from build123d import *

# Parameters (mm, degrees)
SKETCH_1_W                        = 240
SKETCH_1_H                        = 125
EXTRUDE_1_DEPTH                   = 4
HOLE_WIZARD_5_4_5_4_1_D           = 5.4
HOLE_WIZARD_5_4_5_4_1_CSINK_D     = 5.45
HOLE_WIZARD_5_4_5_4_1_CSINK_ANGLE = 90
FILLET_1_R                        = 3
SKETCH_4_R                        = 10
EXTRUDE_2_DEPTH                   = 6
SKETCH_6_W                        = 6.5
SKETCH_6_H                        = 20
EXTRUDE_3_DEPTH                   = 8
SKETCH_7_R                        = 2
CUT_EXTRUDE_1_DEPTH               = 14
FILLET_2_R                        = 4
FILLET_3_R                        = 4
FILLET_4_R                        = 4
EXTRUDE_START                     = 23.5
EXTRUDE_4_DEPTH                   = 8
SKETCH_9_R                        = 5.5
EXTRUDE_5_DEPTH                   = 5
FILLET_5_R                        = 4
FILLET_6_R                        = 4
SKETCH_12_W                       = 7
SKETCH_12_H                       = 8
EXTRUDE_6_DEPTH                   = 20
CUT_EXTRUDE_2_REACH               = 161.108
SKETCH_13_R                       = 2.1
EXTRUDE_7_DEPTH                   = 80
SKETCH_15_R                       = 2.5
EXTRUDE_8_DEPTH                   = 4
EXTRUDE_START_2                   = 15
SKETCH_17_R                       = 2.5
EXTRUDE_9_DEPTH                   = 15


with BuildPart() as part:
    # 草图1 → 凸台-拉伸1 (new body)
    with BuildSketch(Plane(origin=(0, 0, 0), x_dir=(1, 0, 0), z_dir=(0, 1, 0))):
        Rectangle(SKETCH_1_W, SKETCH_1_H)
    extrude(amount=EXTRUDE_1_DEPTH)

    # Ø5.4 (5.4) 直径孔1 (through all)
    with Locations(Plane(origin=(0, 4, 0), x_dir=(1, 0, 0), z_dir=(0, 1, 0))):
        with Locations((112, 54.5), (-112, 54.5), (-112, -54.5), (112, -54.5)):
            CounterSinkHole(HOLE_WIZARD_5_4_5_4_1_D / 2, HOLE_WIZARD_5_4_5_4_1_CSINK_D / 2, counter_sink_angle=HOLE_WIZARD_5_4_5_4_1_CSINK_ANGLE)

    # 圆角1
    fillet_1_edges = [part.edges().sort_by_distance(p)[0] for p in [
        (120, 2, 62.5),
        (-120, 2, 62.5),
        (-120, 2, -62.5),
        (120, 2, -62.5),
    ]]
    fillet(fillet_1_edges, radius=FILLET_1_R)

    # 草图4 → 凸台-拉伸2 (add)
    with BuildSketch(Plane.XY):
        with BuildLine():
            Line((-100, 4), (-46, 4))
            Line((-46, 4), (-46, 36))
            Line((-46, 36), (-73.452041029, 36))
            ThreePointArc((-73.452041029, 36), (-83.25, 40), (-93.047958971, 36))
            Line((-93.047958971, 36), (-100, 36))
            Line((-100, 36), (-100, 4))
        make_face()
        with Locations((-83.25, 26)):
            Circle(SKETCH_4_R, mode=Mode.SUBTRACT)
    extrude(amount=EXTRUDE_2_DEPTH)

    # 草图6 → 凸台-拉伸3 (add)
    with BuildSketch(Plane.XY.offset(6)):
        with Locations((-96.75, 26)):
            Rectangle(SKETCH_6_W, SKETCH_6_H)
        with Locations((-49.25, 26)):
            Rectangle(SKETCH_6_W, SKETCH_6_H)
    extrude(amount=EXTRUDE_3_DEPTH)

    # 草图7 → 切除-拉伸1 (cut)
    with BuildSketch(Plane.XY.offset(14)):
        with Locations((-96.75, 31)):
            Circle(SKETCH_7_R)
        with Locations((-96.75, 21)):
            Circle(SKETCH_7_R)
        with Locations((-49.25, 21)):
            Circle(SKETCH_7_R)
        with Locations((-49.25, 31)):
            Circle(SKETCH_7_R)
    extrude(amount=-CUT_EXTRUDE_1_DEPTH, mode=Mode.SUBTRACT)

    # 圆角2
    fillet_2_edges = [part.edges().sort_by_distance(p)[0] for p in [
        (-49.25, 16, 6),
        (-96.75, 16, 6),
    ]]
    fillet(fillet_2_edges, radius=FILLET_2_R)

    # 圆角3
    fillet_3_edges = [part.edges().sort_by_distance(p)[0] for p in [
        (-73, 4, 6),
    ]]
    fillet(fillet_3_edges, radius=FILLET_3_R)

    # 圆角4
    fillet_4_edges = [part.edges().sort_by_distance(p)[0] for p in [
        (-73, 4, 0),
        (-100, 4, 5),
        (-46, 4, 5),
    ]]
    fillet(fillet_4_edges, radius=FILLET_4_R)

    # 草图8 → 凸台-拉伸4 (add)
    with BuildSketch(Plane(origin=(0, 0, 0), x_dir=(-1, 0, 0), z_dir=(0, 0, -1)).offset(EXTRUDE_START)):
        with BuildLine():
            Line((73, 8), (73, 36))
            ThreePointArc((73, 36), (83.25, 40), (93.5, 36))
            Line((93.5, 36), (93.5, 8))
            Line((93.5, 8), (93.5, 4))
            Line((93.5, 4), (73, 4))
            Line((73, 4), (73, 8))
        make_face()
    extrude(amount=EXTRUDE_4_DEPTH)

    # 草图9 → 凸台-拉伸5 (add)
    with BuildSketch(Plane.XY.offset(-23.5)):
        with Locations((-83.116793534, 25.812971514)):
            Circle(SKETCH_9_R)
    extrude(amount=EXTRUDE_5_DEPTH)

    # 圆角5
    fillet_5_edges = [part.edges().sort_by_distance(p)[0] for p in [
        (-83.25, 4, -31.5),
    ]]
    fillet(fillet_5_edges, radius=FILLET_5_R)

    # 圆角6
    fillet_6_edges = [part.edges().sort_by_distance(p)[0] for p in [
        (-73, 4, -29.5),
        (-83.25, 4, -23.5),
        (-93.5, 4, -29.5),
    ]]
    fillet(fillet_6_edges, radius=FILLET_6_R)

    # 草图12 → 凸台-拉伸6 (add)
    with BuildSketch(Plane(origin=(0, 4, 0), x_dir=(1, 0, 0), z_dir=(0, 1, 0))):
        with Locations((116.5, -30.016568117)):
            Rectangle(SKETCH_12_W, SKETCH_12_H)
        with Locations((69.5, -30.016568117)):
            Rectangle(SKETCH_12_W, SKETCH_12_H)
    extrude(amount=EXTRUDE_6_DEPTH)

    # 草图13 → 切除-拉伸2 (cut, up to next)
    with BuildSketch(Plane.XY.offset(34.016568117), mode=Mode.PRIVATE) as cut_extrude_2_sk1:
        with Locations((69.5, 19)):
            Circle(SKETCH_13_R)
    cut_extrude_2_tool1 = extrude(cut_extrude_2_sk1.sketch, amount=-CUT_EXTRUDE_2_REACH, mode=Mode.PRIVATE) & part.part
    # 草图13 → 切除-拉伸2 (cut, up to next)
    with BuildSketch(Plane.XY.offset(34.016568117), mode=Mode.PRIVATE) as cut_extrude_2_sk2:
        with Locations((69.5, 9)):
            Circle(SKETCH_13_R)
    cut_extrude_2_tool2 = extrude(cut_extrude_2_sk2.sketch, amount=-CUT_EXTRUDE_2_REACH, mode=Mode.PRIVATE) & part.part
    # 草图13 → 切除-拉伸2 (cut, up to next)
    with BuildSketch(Plane.XY.offset(34.016568117), mode=Mode.PRIVATE) as cut_extrude_2_sk3:
        with Locations((116.5, 9)):
            Circle(SKETCH_13_R)
    cut_extrude_2_tool3 = extrude(cut_extrude_2_sk3.sketch, amount=-CUT_EXTRUDE_2_REACH, mode=Mode.PRIVATE) & part.part
    # 草图13 → 切除-拉伸2 (cut, up to next)
    with BuildSketch(Plane.XY.offset(34.016568117), mode=Mode.PRIVATE) as cut_extrude_2_sk4:
        with Locations((116.5, 19)):
            Circle(SKETCH_13_R)
    cut_extrude_2_tool4 = extrude(cut_extrude_2_sk4.sketch, amount=-CUT_EXTRUDE_2_REACH, mode=Mode.PRIVATE) & part.part
    add(cut_extrude_2_tool1.solids().sort_by_distance((69.5, 19, 34.016568))[0], mode=Mode.SUBTRACT)
    add(cut_extrude_2_tool2.solids().sort_by_distance((69.5, 9, 34.016568))[0], mode=Mode.SUBTRACT)
    add(cut_extrude_2_tool3.solids().sort_by_distance((116.5, 9, 34.016568))[0], mode=Mode.SUBTRACT)
    add(cut_extrude_2_tool4.solids().sort_by_distance((116.5, 19, 34.016568))[0], mode=Mode.SUBTRACT)

    # 草图14 → 凸台-拉伸7 (add)
    with BuildSketch(Plane(origin=(0, 4, 0), x_dir=(1, 0, 0), z_dir=(0, 1, 0))):
        with BuildLine():
            Line((109.3, -51.016568117), (96.7, -51.016568117))
            Line((96.7, -51.016568117), (-31.378587674, -51.016568117))
            Line((-31.378587674, -51.016568117), (-31.378587674, 51.016568117))
            Line((-31.378587674, 51.016568117), (95.460915007, 51.016568117))
            Line((95.460915007, 51.016568117), (96.7, 51.016568117))
            Line((96.7, 51.016568117), (109.3, 51.016568117))
            Line((109.3, 51.016568117), (109.3, 54.131727003))
            ThreePointArc((109.3, 54.131727003), (109.275, 54.5), (109.3, 54.868272997))
            Line((109.3, 54.868272997), (109.3, 57.016568117))
            Line((109.3, 57.016568117), (-37.378587674, 57.016568117))
            Line((-37.378587674, 57.016568117), (-37.378587674, -50.764100258))
            Line((-37.378587674, -50.764100258), (-37.378587674, -57.016568117))
            Line((-37.378587674, -57.016568117), (109.3, -57.016568117))
            Line((109.3, -57.016568117), (109.3, -54.868272997))
            ThreePointArc((109.3, -54.868272997), (109.275, -54.5), (109.3, -54.131727003))
            Line((109.3, -54.131727003), (109.3, -51.016568117))
        make_face()
    extrude(amount=EXTRUDE_7_DEPTH)

    # 草图15 → 凸台-拉伸8 (add)
    with BuildSketch(Plane(origin=(0, 0, 51.016568117), x_dir=(-1, 0, 0), z_dir=(0, 0, -1))):
        with Locations((-103, 14)):
            Circle(SKETCH_15_R)
    extrude(amount=EXTRUDE_8_DEPTH)

    # 草图17 → 凸台-拉伸9 (add)
    with BuildSketch(Plane.XY.offset(-51.016568117).offset(EXTRUDE_START_2)):
        with Locations(Location((103, 14, 0), (0, 0, 180))):
            Circle(SKETCH_17_R)
    extrude(amount=-EXTRUDE_9_DEPTH)


solid = part.part
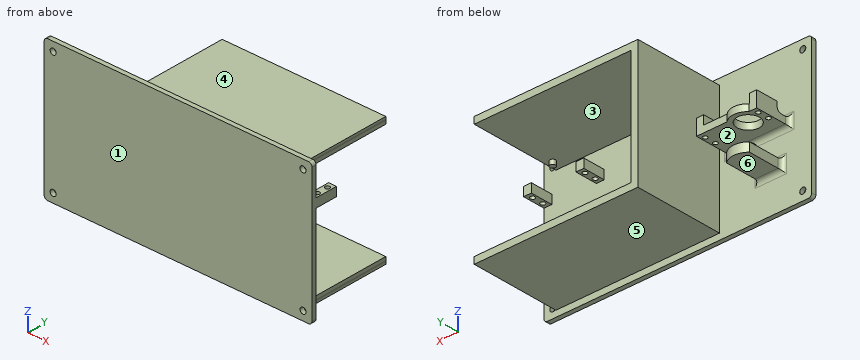
Part model, mm, in its own coordinate system. Face numbers are marked on the shaded views. A direction names the side the tool comes from. Give positions to 0.01 mm unless a question says otherwise; leave off trailing zeros. Loops run counter-clockwise (first coordinate to the right, second up) from the corner with the lowest first, then second, coordinate; pieces in that order, holes last. Notation, with made-up numbers: M -8,-21 L 27,-21 A22 ccw 27,-4 Z; hole C -3,73.25 d6. An arc over 180 degrees is marked long. Put each result on its own line as item: value. Start each with the question number.
1) Saw through at C-C (x = 31). List the corners of the cut face in (y, z), then the cut area to 3 significant figures.
2) Flat gauge pins, fed straight in: pin 1 (4 mm diameter, centred on y = 18, z = -27, fed in from -X); pin 2 (8 mm diameter, centred on y = 54, z = 10, fed in from -X); pin 3 (5 mm diameter, centred on x = -58.5, y = 39, fed in from -Z) (3 decimals); pin 4 (16 mm diameter, centred on x = -77.5, y = 20, fed in from -Z). Where does each tip first touch, or does it go through?
3) Pull direction Z, two halves, no side cores. Call the marked faces 1, 2, 3 and 4: +Z half, -Z half, draft (parallel to the pull), parting line (faces both ways), or undercut.
4) Probe probe 1 along Y at (x, z) = (116.5, 28); probe 2 along Z at (x, y) = (112, 2); probe 3 along Y at (x, z) = (-49, 4). List the from-to ranges inside material, lowest first.
5) Saw through at B-B (y = 63.5). List the corners of the cut face in (x, z) (3 decimals), then the cut area to 3 significant figures.
6) 3-axis set-ups, long thin cutter, end or side, ignore diameter. For the marked faces 5 and 6: which of +Z, -Z, +X, -X, +Y, -Y reach the whole face in a straight line?
7) Saw through at A-A (x = -112). List the corners of the cut face in (y, z) (3 decimals).
8) Saw through at D-D (x = 103). List the corners of the cut face in (y, z).
Numbers:
1. outline: M 0,-62.5 L 4,-62.5 L 4,-57.02 L 84,-57.02 L 84,-51.02 L 4,-51.02 L 4,51.02 L 84,51.02 L 84,57.02 L 4,57.02 L 4,62.5 L 0,62.5 Z
1. area: 1,460 mm^2
2. pin 1: x = -93.5
2. pin 2: x = -37.38
2. pin 3: through
2. pin 4: z = -31.5
3. face 1: draft
3. face 2: undercut
3. face 3: undercut
3. face 4: +Z half
4. probe 1: 0 to 6.9, 11.1 to 16.9, 21.1 to 24
4. probe 2: -62.5 to -57.2, -51.8 to 51.8, 57.2 to 62.5
4. probe 3: 0 to 19.02, 22.98 to 29.02, 32.98 to 36
5. outline: M -37.379,-57.017 L 109.3,-57.017 L 109.3,-54.868 A2.725 cw 109.3,-54.132 L 109.3,-51.017 L -31.379,-51.017 L -31.379,51.017 L 109.3,51.017 L 109.3,54.132 A2.725 cw 109.3,54.868 L 109.3,57.017 L -37.379,57.017 Z
5. area: 2,370 mm^2
6. face 5: -Z, +X, -X, +Y
6. face 6: -Z, -X, +Y
7. outline: M 0,-62.5 L 4,-62.5 L 4,-57.225 L 3.975,-57.2 L 0,-57.2 Z; M 0,-51.8 L 3.975,-51.8 L 4,-51.775 L 4,51.775 L 3.975,51.8 L 0,51.8 Z; M 0,57.2 L 3.975,57.2 L 4,57.225 L 4,62.5 L 0,62.5 Z
8. outline: M 0,-62.5 L 4,-62.5 L 4,-57.02 L 84,-57.02 L 84,-51.02 L 16.5,-51.02 L 16.5,-36.02 L 11.5,-36.02 L 11.5,-51.02 L 4,-51.02 L 4,51.02 L 11.5,51.02 L 11.5,47.02 L 16.5,47.02 L 16.5,51.02 L 84,51.02 L 84,57.02 L 4,57.02 L 4,62.5 L 0,62.5 Z
